```python
from build123d import *

# Parameters (mm, degrees)
BOSS_EXTRUDE1_DEPTH     = 22
BOSS_EXTRUDE2_DEPTH     = 36
BOSS_EXTRUDE3_DEPTH     = 46
SKETCH4_W               = 8
SKETCH4_H               = 3.5
CUT_EXTRUDE1_DEPTH      = 61.012155958
CUT_EXTRUDE3_DEPTH      = 11
CUT_EXTRUDE3_DEPTH_BACK = 11
BOSS_EXTRUDE4_DEPTH     = 4
LPATTERN1_COUNT         = 7
LPATTERN1_PITCH         = 8


with BuildPart() as part:
    # Sketch1 → Boss-Extrude1 (new body)
    with BuildSketch(Plane.XY):
        with BuildLine():
            Line((-69.282032303, -10), (-43.874821937, -10))
            ThreePointArc((-43.874821937, -10), (-45, 0), (-43.874821937, 10))
            Line((-43.874821937, 10), (-69.282032303, 10))
            ThreePointArc((-69.282032303, 10), (-70, 0), (-69.282032303, -10))
        make_face()
    extrude(amount=BOSS_EXTRUDE1_DEPTH)

    # Sketch1<3> → Boss-Extrude2 (add)
    with BuildSketch(Plane.XY):
        with BuildLine():
            Line((-43.874821937, -10), (-22.912878475, -10))
            ThreePointArc((-22.912878475, -10), (-25, 0), (-22.912878475, 10))
            Line((-22.912878475, 10), (-43.874821937, 10))
            ThreePointArc((-43.874821937, 10), (-45, 0), (-43.874821937, -10))
        make_face()
    extrude(amount=BOSS_EXTRUDE2_DEPTH)

    # Sketch1<4> → Boss-Extrude3 (add)
    with BuildSketch(Plane.XY):
        with BuildLine():
            Line((-22.912878475, -10), (-13.282032303, -10))
            Line((-13.282032303, -10), (-9.987844042, -0.827246844))
            ThreePointArc((-9.987844042, -0.827246844), (-10.021711204, -0.081673003), (-10, 0.664353779))
            Line((-10, 0.664353779), (-13.282032303, 10))
            Line((-13.282032303, 10), (-22.912878475, 10))
            ThreePointArc((-22.912878475, 10), (-25, 0), (-22.912878475, -10))
        make_face()
    extrude(amount=BOSS_EXTRUDE3_DEPTH)

    # Sketch4 → Cut-Extrude1 (cut, through all)
    with BuildSketch(Plane.ZY.offset(70)):
        with Locations((18, 8.25)):
            Rectangle(SKETCH4_W, SKETCH4_H)
        with Locations((18, -8.25)):
            Rectangle(SKETCH4_W, SKETCH4_H)
    extrude(amount=-CUT_EXTRUDE1_DEPTH, mode=Mode.SUBTRACT)

    # Sketch8 → Cut-Extrude3 (cut, two sides)
    with BuildSketch(Plane(origin=(0, 0, 0), x_dir=(1, 0, 0), z_dir=(0, 1, 0))) as cut_extrude3_sk:
        Polygon((-13.282032303, -7), (-9.987844042, -10.294188261), (-9.987844042, 0), (-13.282032303, 0), align=None)
    extrude(amount=CUT_EXTRUDE3_DEPTH, mode=Mode.SUBTRACT)
    extrude(cut_extrude3_sk.sketch, amount=-CUT_EXTRUDE3_DEPTH_BACK, mode=Mode.SUBTRACT)

    # Sketch7 → Boss-Extrude4 (add)
    with BuildSketch(Plane(origin=(0, 0, 0), x_dir=(-1, 0, 0), z_dir=(0, 0, -1))):
        with BuildLine():
            Line((14, 10), (14, -10))
            Line((14, -10), (14.966629547, -10))
            ThreePointArc((14.966629547, -10), (18, 0), (14.966629547, 10))
            Line((14.966629547, 10), (14, 10))
        make_face()
    boss_extrude4 = extrude(amount=BOSS_EXTRUDE4_DEPTH)

    # LPattern1: Boss-Extrude4 ×7
    with Locations(*[(-i * LPATTERN1_PITCH, 0, 0) for i in range(1, LPATTERN1_COUNT)]):
        add(boss_extrude4)


solid = part.part
```
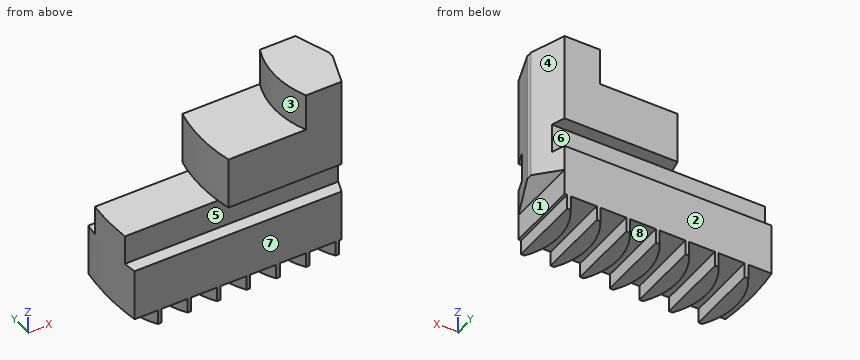
Design review of the part built by this model. Coordinates are the model's own, in mm. Face numbers are marked on the shaded views. A direction names the side the tool comes from. Give positions to 0.01 mm unless a question says otherwise; leave off trailing zeros. Write each loop counter-clockwise with the first axis right and the second up, starting at its lowest first coordinate (ties: lowest second). Pieces come first, ordered by that corner, then holes.
(1) Add section D-D (z = 13). Give the boundary of the cut face in (x, y).
Checked values:
outline: (-69.28, -10) - (-13.28, -10) - (-9.99, -0.83) arc R10.02 cw to (-10, 0.66) - (-13.28, 10) - (-69.28, 10) arc R70 ccw to start
(2) Add section C-C (x = -19). Give the boundary of the cut face in (y, z).
Checked values:
outline: (-10, 0) - (10, 0) - (10, 14) - (6.5, 14) - (6.5, 22) - (10, 22) - (10, 46) - (-10, 46) - (-10, 22) - (-6.5, 22) - (-6.5, 14) - (-10, 14) - close
(3) Tool access review of the marked faces 1, 2, 3, 4 and 5: name each direction out of +Z, -Z, +X, -X, +Y, -Y from which nothing blocks a thin tool from reaching the whole face with its end or side.
Checked values:
face 1: -Z, +X, +Y, -Y
face 2: +Z, -Z, +X, -X, +Y
face 3: +Z, -X
face 4: +Z, -Z, +X, +Y
face 5: +X, -X, -Y
(4) Add section B-B (z = 26.5). Give the boundary of the cut face in (x, y), and give its area (3 significant figures).
Checked values:
outline: (-43.87, -10) - (-13.28, -10) - (-9.99, -0.83) arc R10.02 cw to (-10, 0.66) - (-13.28, 10) - (-43.87, 10) arc R45 ccw to start
area: 662 mm2
(5) Wall thickness on line 1 along Z through (x, y) = (-41.5, -6.75); line 2 along Z through (x, y) = (-34.5, 5.5); line 3 along Z through (x, y) = (-64.5, 2.5): over which ranges is each line inside the solid? List them lowest first.
Checked values:
line 1: z = 0 to 14, 22 to 36
line 2: z = 0 to 36
line 3: z = -4 to 22
(6) Mouldability with a two-part tool opening along Z and no side actions: class the marked faces 6, 7 and 8 as +Z half, -Z half, draft (parallel to the pull), parting line (faces both ways), or undercut.
Checked values:
face 6: undercut
face 7: draft
face 8: -Z half
(7) Clearance check with flat-ended pins moving along their axes: pin 1 Ø5 at (x, y) = (-25.5, -8) entering from +Z; pin 2 Ø4.5 at (y, z) = (-4, -2) entering from +X; pin 3 Ø6 at (x, z) = (-34.5, 18.5) entering from -Y; pin 4 Ø6 at (x, y) = (-49, -7) entering from +Z. State where each tip first meets the part, or that it passes through.
Checked values:
pin 1: stops at z = 46
pin 2: stops at x = -13.28
pin 3: stops at y = -6.5
pin 4: stops at z = 22
(8) Add section A-A (x = -52). Give the boundary of the cut face in (y, z).
Checked values:
outline: (-10, 0) - (10, 0) - (10, 14) - (6.5, 14) - (6.5, 22) - (-6.5, 22) - (-6.5, 14) - (-10, 14) - close
